from build123d import *

# Parameters (mm, degrees)
SKETCH1_R           = 3.175
BOSS_EXTRUDE1_DEPTH = 0.635
CUT_EXTRUDE1_START  = -0.635
CUT_EXTRUDE1_DEPTH  = 1.27
CUT_EXTRUDE2_DEPTH  = 37.222840302


# Read off the part's stored shape, not the designer's step: Cut-Extrude1
with BuildPart() as part:
    # Sketch1 → Boss-Extrude1 (new, symmetric)
    with BuildSketch(Plane.XY):
        with BuildLine():
            Line((-9.484545184, 0.876942223), (-12.7, -33.89972345))
            Line((-12.7, -33.89972345), (12.7, -33.89972345))
            Line((12.7, -33.89972345), (9.484545184, 0.876942223))
            ThreePointArc((9.484545184, 0.876942223), (0, 9.525), (-9.484545184, 0.876942223))
        make_face()
        Circle(SKETCH1_R, mode=Mode.SUBTRACT)
    extrude(amount=BOSS_EXTRUDE1_DEPTH, both=True)

    # Cut-Extrude1 outline → Cut-Extrude1 (cut)
    with BuildSketch(Plane.XY.offset(CUT_EXTRUDE1_START)):
        with BuildLine():
            Line((-8.497954961, -33.89972345), (8.76063713, -33.89972345))
            add(Edge.make_bspline(
                [(8.76063713, -33.89972345), (0.306373234, -25.111661594), (-8.497954961, -33.89972345)],
                knots=[2.496380088, 2.496380088, 2.496380088, 3.988409978, 3.988409978, 3.988409978], degree=2, weights=[1, 0.73439942, 1]))
        make_face()
    extrude(amount=CUT_EXTRUDE1_DEPTH, mode=Mode.SUBTRACT)

    # Sketch3 → Cut-Extrude2 (cut, through all)
    with BuildSketch(Plane.XY.offset(0.635)):
        with BuildLine():
            Line((8.76063713, -33.89972345), (12.7, -33.89972345))
            Line((12.7, -33.89972345), (12.314154974, -29.726626876))
            ThreePointArc((12.314154974, -29.726626876), (10.7009799, -32.790811849), (7.245953049, -32.557674927))
            add(Edge.make_bspline(
                [(8.76063713, -33.89972345), (8.051791445, -33.162890557), (7.245953049, -32.557674927)],
                knots=[2.496380088, 2.496380088, 2.496380088, 2.651046381, 2.651046381, 2.651046381], degree=2, weights=[1, 0.997011282, 1]))
        make_face()
        with BuildLine():
            Line((-12.7, -33.89972345), (-8.497954961, -33.89972345))
            add(Edge.make_bspline(
                [(-7.23241505, -32.785101753), (-7.896265785, -33.299145918), (-8.497954961, -33.89972345)],
                knots=[3.862260272, 3.862260272, 3.862260272, 3.988409978, 3.988409978, 3.988409978], degree=2, weights=[1, 0.998011441, 1]))
            ThreePointArc((-7.23241505, -32.785101753), (-10.704172961, -33.057927648), (-12.337805101, -29.982414196))
            Line((-12.337805101, -29.982414196), (-12.7, -33.89972345))
        make_face()
    extrude(amount=-CUT_EXTRUDE2_DEPTH, mode=Mode.SUBTRACT)


solid = part.part
The listing builds one solid part. Answer for the finished solid, in the listing's coordinates (mm). Give positions to 0.01 mm unless a question says otherwise; leave off trailing zeros. Order: outer loops, then holes, each group sorted by start corner. A loop starts at its lowest first (then second) coordinate and runs counter-clockwise, first axis right, second up. Notation, with made-up numbers: (0, -13.5) -> (31, -13.5) arc R16 cw to (31, 14.5) -> close; hole circle Ø11 at (-20, 10). An arc over 180 degrees is marked (long way). Put each result on its own line as item: value.
Item 1: Given P1, Ø10, axis at x = 0, y = 0, coming from the -Z side (3 decimals), flat-ended and moving along its own axis, determine where the tip first touches the part or whether it passes through.
Established:
P1: stops at z = -0.635
Item 2: A cutting plane is placed at B-B on y = -21. Give the vertices of the cut face in (x, z) (3 decimals).
Established:
outline: (-11.507, -0.635) -> (11.507, -0.635) -> (11.507, 0.635) -> (-11.507, 0.635) -> close
Item 3: For a pull along Y with two mould halves and no side action, classify faces 1 (the face through (0, -12, -0.635)), 2 (the face through (10.92, -14.64, 0.01)), 3 (the face through (-0.69, -3.1, -0.01)) as released by +Y, released by -Y, zero draft, split by the parting line, or undercut.
Established:
face 1: zero draft
face 2: released by +Y
face 3: undercut
Item 4: Straight lines are drawn through the part: line 1 (Y direction, x = 0, z = 0.25) (3 decimals); line 2 (Y direction, x = 4.25, z = 0.35); line 3 (X direction, y = -16.5, z = 0.4). For each, find the intervals that lie inside material, in ascending order.
Established:
line 1: y = -30.18 to -3.175, 3.175 to 9.525
line 2: y = -30.91 to 8.52
line 3: x = -11.09 to 11.09
Item 5: A cutting plane is placed at A-A on y = 0. Give the vertices of the cut face in (x, z) (3 decimals).
Established:
outline: (-9.566, -0.635) -> (-3.175, -0.635) -> (-3.175, 0.635) -> (-9.566, 0.635) -> close; (3.175, -0.635) -> (9.566, -0.635) -> (9.566, 0.635) -> (3.175, 0.635) -> close
Item 6: A cutting plane is placed at C-C on x = -9. Give the vertices of the cut face in (y, z) (3 decimals), plus the area to 3 significant figures.
Established:
outline: (-33.445, -0.635) -> (3.119, -0.635) -> (3.119, 0.635) -> (-33.445, 0.635) -> close
area: 46.4 mm^2
